Could you check a few things on this model? Use its own coordinates, in mm. Face numbers are marked on the shaded views. A direction names the side the tool comes from. Give positions to 0.01 mm unless a question says otherwise; leave off trailing zeros. Loops run counter-clockwise (first coordinate to the right, second up) from the corner with the lowest first, then second, coordinate; pieces in that order, holes last. Notation, with made-up numbers: (51, 84) - (64, 84) arc R27 cw to (64, 100) - close; hole circle Ø10 at (64.5, 3.5). An arc over 180 degrees is marked (long way). Write each question's results on one line, items separated by ' | '. Start each with the question number.
(1) Suppose I cut it at A-A (y = 4.5). Please give me the cut outline in (x, z), and give its area (4 significant figures).
(2) Suppose I cut it at B-B (z = 16.25). Please give me the cut outline in (x, y), and give its area (3 significant figures).
(3) On a 3-axis mill with a long thin cutter (end or side, diameter ignored), from which of +Z, -Z, +X, -X, +Y, -Y can I reach the whole of each face in a straight line? I mean the marked faces 1 and 2. Say none if no direction works.
(4) Suppose I cut it at C-C (y = 29.5). Please give me the cut outline in (x, z).
(5) For pin 1 (1.5 mm diameter, centred on y = 26, z = 14.5, fed in from -X); pin 2 (4.5 mm diameter, centred on y = 47, z = 15.5, fed in from +X); pin 3 (9 mm diameter, centred on y = 29.5, z = 7, fed in from +X), each with a flat end and sliding along its axis, tell me the tip position at first contact or that it passes through.
(6) I need wall thicknesses on line 1 (Y direction, x = 0.7, z = 7); line 2 (Y direction, x = 2.45, z = 7); line 3 (X direction, y = 51, z = 15). Which ranges of each line are inside material? Lowest first, please.
from build123d import *

# Parameters (mm, degrees)
SKETCH1_W                                        = 30
SKETCH1_H                                        = 63
BOSS_EXTRUDE1_DEPTH                              = 4
SKETCH2_R                                        = 5
CUT_EXTRUDE1_DEPTH                               = 70.89277502
F_4_0_4_DIAMETER_HOLE1_D                         = 4
SKETCH12_W                                       = 14.5
SKETCH12_H                                       = 24
CUT_EXTRUDE2_DEPTH                               = 70.89277502
SKETCH13_W                                       = 42.673617324
SKETCH13_H                                       = 65.779819875
CUT_EXTRUDE5_DEPTH                               = 4
F_4_0_4_DIAMETER_HOLE6_D                         = 4
CBORE_FOR_M3_PAN_HEAD_MACHINE_SCREW7_D           = 3.2
CBORE_FOR_M3_PAN_HEAD_MACHINE_SCREW7_CBORE_D     = 9
CBORE_FOR_M3_PAN_HEAD_MACHINE_SCREW7_CBORE_DEPTH = 1
CSK_FOR_M3_FLAT_HEAD_MACHINE_SCREW1_D            = 3.2
CSK_FOR_M3_FLAT_HEAD_MACHINE_SCREW1_CSINK_D      = 4
CSK_FOR_M3_FLAT_HEAD_MACHINE_SCREW1_CSINK_ANGLE  = 90
CUT_EXTRUDE6_DEPTH                               = 70.89277502
CUT_EXTRUDE6_DEPTH_BACK                          = 70.89277502
SKETCH45_W                                       = 4
SKETCH45_H                                       = 39
SKETCH46_W                                       = 0.1
SKETCH46_H                                       = 63
CUT_EXTRUDE7_DEPTH                               = 69.271516755
BOSS_EXTRUDE2_START                              = -1.4
SKETCH47_R                                       = 5
SKETCH47_R_2                                     = 3.5
BOSS_EXTRUDE2_DEPTH                              = 1.4


with BuildPart() as part:
    # Sketch1 → Boss-Extrude1 (new body)
    with BuildSketch(Plane(origin=(0, 0, 0), x_dir=(0, 0, -1), z_dir=(1, 0, 0))):
        with Locations((-15, 31.5)):
            Rectangle(SKETCH1_W, SKETCH1_H)
    boss_extrude1 = extrude(amount=-BOSS_EXTRUDE1_DEPTH)

    # Sketch2 → Cut-Extrude1 (cut, through all)
    with BuildSketch(Plane(origin=(0, 0, 0), x_dir=(0, 0, -1), z_dir=(1, 0, 0))):
        with Locations((-7, 29.5)):
            Circle(SKETCH2_R)
    cut_extrude1 = extrude(amount=-CUT_EXTRUDE1_DEPTH, mode=Mode.SUBTRACT)

    # Ø4.0 (4) Diameter Hole1 (through all)
    with Locations(Plane(origin=(0, 4.5, 7), x_dir=(0, 0, 1), z_dir=(1, 0, 0))):
        with Locations((0, 0)):
            Hole(F_4_0_4_DIAMETER_HOLE1_D / 2)

    # Sketch12 → Cut-Extrude2 (cut, through all)
    with BuildSketch(Plane(origin=(0, 0, 0), x_dir=(0, 0, -1), z_dir=(1, 0, 0))):
        with Locations((-22.75, 12)):
            Rectangle(SKETCH12_W, SKETCH12_H)
    cut_extrude2 = extrude(amount=-CUT_EXTRUDE2_DEPTH, mode=Mode.SUBTRACT)

    # Mirror7: Boss-Extrude1, Cut-Extrude1, Cut-Extrude2 across plane
    add(boss_extrude1.mirror(Plane(origin=(0, 0, 0), x_dir=(0, 0, 1), z_dir=(1, 0, 0))))
    add(cut_extrude1.mirror(Plane(origin=(0, 0, 0), x_dir=(0, 0, 1), z_dir=(1, 0, 0))), mode=Mode.SUBTRACT)
    add(cut_extrude2.mirror(Plane(origin=(0, 0, 0), x_dir=(0, 0, 1), z_dir=(1, 0, 0))), mode=Mode.SUBTRACT)

    # Sketch13 → Cut-Extrude5 (cut)
    with BuildSketch(Plane.ZY.offset(4)):
        with Locations((15.520409967, 30.110090063)):
            Rectangle(SKETCH13_W, SKETCH13_H)
    extrude(amount=-CUT_EXTRUDE5_DEPTH, mode=Mode.SUBTRACT)

    # Ø4.0 (4) Diameter Hole6 (through all)
    with Locations(Plane(origin=(0, 4.5, 7), x_dir=(0, 0, -1), z_dir=(-1, 0, 0))):
        with Locations((0, 0)):
            Hole(F_4_0_4_DIAMETER_HOLE6_D / 2)

    # CBORE for M3 Pan Head Machine Screw7 (through all)
    with Locations(Plane(origin=(4, 47.360571099, 16), x_dir=(0, 0, 1), z_dir=(1, 0, 0))):
        with Locations((0, 0)):
            CounterBoreHole(CBORE_FOR_M3_PAN_HEAD_MACHINE_SCREW7_D / 2, CBORE_FOR_M3_PAN_HEAD_MACHINE_SCREW7_CBORE_D / 2, CBORE_FOR_M3_PAN_HEAD_MACHINE_SCREW7_CBORE_DEPTH)

    # CSK for M3 Flat Head Machine Screw1 (through all)
    with Locations(Plane(origin=(0, 36.032608687, 19.33966579), x_dir=(0, 0, -1), z_dir=(-1, 0, 0))):
        with Locations((0, 0), (14.431341448, -7.272)):
            CounterSinkHole(CSK_FOR_M3_FLAT_HEAD_MACHINE_SCREW1_D / 2, CSK_FOR_M3_FLAT_HEAD_MACHINE_SCREW1_CSINK_D / 2, counter_sink_angle=CSK_FOR_M3_FLAT_HEAD_MACHINE_SCREW1_CSINK_ANGLE)

    # Sketch45 → Cut-Extrude6 (cut, two sides: drawn at the far end of the back side and taken through both)
    with BuildSketch(Plane(origin=(4, 0, 0), x_dir=(0, 0, -1), z_dir=(1, 0, 0)).offset(-CUT_EXTRUDE6_DEPTH_BACK)):
        with Locations((-28, 43.5)):
            Rectangle(SKETCH45_W, SKETCH45_H)
    extrude(amount=CUT_EXTRUDE6_DEPTH + CUT_EXTRUDE6_DEPTH_BACK, mode=Mode.SUBTRACT)

    # Sketch46 → Cut-Extrude7 (cut, through all)
    with BuildSketch(Plane(origin=(0, 0, 0), x_dir=(-1, 0, 0), z_dir=(0, 0, -1))):
        with Locations((-3.95, 31.5)):
            Rectangle(SKETCH46_W, SKETCH46_H)
    extrude(amount=-CUT_EXTRUDE7_DEPTH, mode=Mode.SUBTRACT)

    # Sketch47 → Boss-Extrude2 (add)
    with BuildSketch(Plane.ZY.offset(BOSS_EXTRUDE2_START)):
        with Locations(Location((7, 29.5, 0), (0, 0, 270))):
            Circle(SKETCH47_R)
        with Locations((7, 29.5)):
            Circle(SKETCH47_R_2, mode=Mode.SUBTRACT)
    extrude(amount=BOSS_EXTRUDE2_DEPTH)


solid = part.part
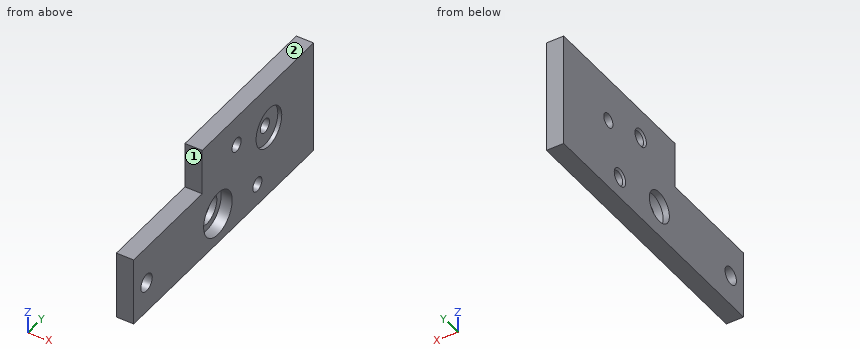
Output values:
1) outline: (0, 0) - (3.9, 0) - (3.9, 5) - (0, 5) - close; (0, 9) - (3.9, 9) - (3.9, 15.5) - (0, 15.5) - close | area: 44.85 mm2
2) outline: (0, 24) - (3.9, 24) - (3.9, 42.87) - (3, 42.87) - (3, 45.78) - (0, 45.78) - close; (0, 48.94) - (3, 48.94) - (3, 51.85) - (3.9, 51.85) - (3.9, 63) - (0, 63) - close | area: 135 mm2
3) face 1: +Z, +X, -X, -Y | face 2: +Z, +X, -X, +Y, -Y
4) outline: (0, 0) - (3.9, 0) - (3.9, 2) - (1.4, 2) - (1.4, 3.5) - (0, 3.5) - close; (0, 10.5) - (1.4, 10.5) - (1.4, 12) - (3.9, 12) - (3.9, 26) - (0, 26) - close
5) pin 1: x = 0 | pin 2: x = 3 | pin 3: x = 1.4
6) line 1: 0 to 2.5, 6.5 to 26, 33 to 63 | line 2: 0 to 2.5, 6.5 to 24.5, 34.5 to 63 | line 3: 0 to 3
